Build history of the part. All positions in model axes, mm. A direction names the side the tool comes from. Round coordinates to 2 decimals unless told otherwise and drop trailing zeros. Order: outer loops, then holes, each group sorted by start corner. A loop starts at its lowest first (then second) coordinate and runs counter-clockwise, first axis right, second up. Notation, with made-up numbers: (-38, 37.25) -> (-17, 37.25) arc R21 cw to (-17, 68.25) -> close; hole circle Ø10 at (30.25, 57.25). An arc over 180 degrees is marked (long way). Write item = value, one per line.
from build123d import *

# Parameters (mm, degrees)
EXTRUDE_3_DEPTH = 10
EXTRUDE_START   = -12
EXTRUDE_4_DEPTH = 2
EXTRUDE_START_2 = 1
EXTRUDE_5_DEPTH = 1
SKETCH_2_R      = 5
SKETCH_2_R_2    = 3.5
EXTRUDE_6_DEPTH = 8
SKETCH_2_2_R    = 3.5
EXTRUDE_7_DEPTH = 7


# Read off the part's stored shape, not the designer's step: 凸台-拉伸4
with BuildPart() as part:
    # 草图1 → 凸台-拉伸3 (new body)
    with BuildSketch(Plane(origin=(0, 0, 0), x_dir=(1, 0, 0), z_dir=(0, 1, 0))):
        with BuildLine():
            Line((-8.229462415, 6.472103102), (-9.229462415, 7.472103102))
            ThreePointArc((-9.229462415, 7.472103102), (-9.371981305, 6.954608621), (-9.42, 6.42))
            Line((-9.42, 6.42), (-9.42, -6.42))
            ThreePointArc((-9.42, -6.42), (-9.371981305, -6.954608621), (-9.229462415, -7.472103102))
            Line((-9.229462415, -7.472103102), (-8.229462415, -6.472103102))
            ThreePointArc((-8.229462415, -6.472103102), (-8.371981305, -5.954608621), (-8.42, -5.42))
            Line((-8.42, -5.42), (-8.42, 5.42))
            ThreePointArc((-8.42, 5.42), (-8.371981305, 5.954608621), (-8.229462415, 6.472103102))
        make_face()
        with BuildLine():
            Line((-6.472103102, 8.229462415), (-7.472103102, 9.229462415))
            ThreePointArc((-7.472103102, 9.229462415), (-8.541320344, 8.541320344), (-9.229462415, 7.472103102))
            Line((-9.229462415, 7.472103102), (-8.229462415, 6.472103102))
            ThreePointArc((-8.229462415, 6.472103102), (-7.541320344, 7.541320344), (-6.472103102, 8.229462415))
        make_face()
        with BuildLine():
            ThreePointArc((7.472103102, 9.229462415), (6.954608621, 9.371981305), (6.42, 9.42))
            Line((6.42, 9.42), (-6.42, 9.42))
            ThreePointArc((-6.42, 9.42), (-6.954608621, 9.371981305), (-7.472103102, 9.229462415))
            Line((-7.472103102, 9.229462415), (-6.472103102, 8.229462415))
            ThreePointArc((-6.472103102, 8.229462415), (-5.954608621, 8.371981305), (-5.42, 8.42))
            Line((-5.42, 8.42), (5.42, 8.42))
            ThreePointArc((5.42, 8.42), (5.954608621, 8.371981305), (6.472103102, 8.229462415))
            Line((6.472103102, 8.229462415), (7.472103102, 9.229462415))
        make_face()
        with BuildLine():
            Line((-8.229462415, -6.472103102), (-9.229462415, -7.472103102))
            ThreePointArc((-9.229462415, -7.472103102), (-8.541320344, -8.541320344), (-7.472103102, -9.229462415))
            Line((-7.472103102, -9.229462415), (-6.472103102, -8.229462415))
            ThreePointArc((-6.472103102, -8.229462415), (-7.541320344, -7.541320344), (-8.229462415, -6.472103102))
        make_face()
        with BuildLine():
            ThreePointArc((6.42, -9.42), (6.954608621, -9.371981305), (7.472103102, -9.229462415))
            Line((7.472103102, -9.229462415), (6.472103102, -8.229462415))
            ThreePointArc((6.472103102, -8.229462415), (5.954608621, -8.371981305), (5.42, -8.42))
            Line((5.42, -8.42), (-5.42, -8.42))
            ThreePointArc((-5.42, -8.42), (-5.954608621, -8.371981305), (-6.472103102, -8.229462415))
            Line((-6.472103102, -8.229462415), (-7.472103102, -9.229462415))
            ThreePointArc((-7.472103102, -9.229462415), (-6.954608621, -9.371981305), (-6.42, -9.42))
            Line((-6.42, -9.42), (6.42, -9.42))
        make_face()
        with BuildLine():
            ThreePointArc((7.472103102, -9.229462415), (8.541320344, -8.541320344), (9.229462415, -7.472103102))
            Line((9.229462415, -7.472103102), (8.229462415, -6.472103102))
            ThreePointArc((8.229462415, -6.472103102), (7.541320344, -7.541320344), (6.472103102, -8.229462415))
            Line((6.472103102, -8.229462415), (7.472103102, -9.229462415))
        make_face()
        with BuildLine():
            ThreePointArc((9.42, 6.42), (9.371981305, 6.954608621), (9.229462415, 7.472103102))
            Line((9.229462415, 7.472103102), (8.229462415, 6.472103102))
            ThreePointArc((8.229462415, 6.472103102), (8.371981305, 5.954608621), (8.42, 5.42))
            Line((8.42, 5.42), (8.42, -5.42))
            ThreePointArc((8.42, -5.42), (8.371981305, -5.954608621), (8.229462415, -6.472103102))
            Line((8.229462415, -6.472103102), (9.229462415, -7.472103102))
            ThreePointArc((9.229462415, -7.472103102), (9.371981305, -6.954608621), (9.42, -6.42))
            Line((9.42, -6.42), (9.42, 6.42))
        make_face()
        with BuildLine():
            ThreePointArc((9.229462415, 7.472103102), (8.541320344, 8.541320344), (7.472103102, 9.229462415))
            Line((7.472103102, 9.229462415), (6.472103102, 8.229462415))
            ThreePointArc((6.472103102, 8.229462415), (7.541320344, 7.541320344), (8.229462415, 6.472103102))
            Line((8.229462415, 6.472103102), (9.229462415, 7.472103102))
        make_face()
    extrude(amount=-EXTRUDE_3_DEPTH)

    # 凸台-拉伸4 outline → 凸台-拉伸4 (add)
    with BuildSketch(Plane(origin=(0, 0, 0), x_dir=(1, 0, 0), z_dir=(0, 1, 0)).offset(EXTRUDE_START)):
        with BuildLine():
            Line((-9.42, 6.42), (-9.42, -6.42))
            ThreePointArc((-9.42, -6.42), (-8.541320344, -8.541320344), (-6.42, -9.42))
            Line((-6.42, -9.42), (6.42, -9.42))
            ThreePointArc((6.42, -9.42), (8.541320344, -8.541320344), (9.42, -6.42))
            Line((9.42, -6.42), (9.42, 6.42))
            ThreePointArc((9.42, 6.42), (8.541320344, 8.541320344), (6.42, 9.42))
            Line((6.42, 9.42), (-6.42, 9.42))
            ThreePointArc((-6.42, 9.42), (-8.541320344, 8.541320344), (-9.42, 6.42))
        make_face()
    extrude(amount=EXTRUDE_4_DEPTH)

    # 草图1<7> → 凸台-拉伸5 (add)
    with BuildSketch(Plane(origin=(0, 0, 0), x_dir=(1, 0, 0), z_dir=(0, 1, 0)).offset(EXTRUDE_START_2)):
        with BuildLine():
            Line((-8.229462415, 6.472103102), (-9.229462415, 7.472103102))
            ThreePointArc((-9.229462415, 7.472103102), (-9.371981305, 6.954608621), (-9.42, 6.42))
            Line((-9.42, 6.42), (-9.42, -6.42))
            ThreePointArc((-9.42, -6.42), (-9.371981305, -6.954608621), (-9.229462415, -7.472103102))
            Line((-9.229462415, -7.472103102), (-8.229462415, -6.472103102))
            ThreePointArc((-8.229462415, -6.472103102), (-8.371981305, -5.954608621), (-8.42, -5.42))
            Line((-8.42, -5.42), (-8.42, 5.42))
            ThreePointArc((-8.42, 5.42), (-8.371981305, 5.954608621), (-8.229462415, 6.472103102))
        make_face()
        with BuildLine():
            ThreePointArc((7.472103102, 9.229462415), (6.954608621, 9.371981305), (6.42, 9.42))
            Line((6.42, 9.42), (-6.42, 9.42))
            ThreePointArc((-6.42, 9.42), (-6.954608621, 9.371981305), (-7.472103102, 9.229462415))
            Line((-7.472103102, 9.229462415), (-6.472103102, 8.229462415))
            ThreePointArc((-6.472103102, 8.229462415), (-5.954608621, 8.371981305), (-5.42, 8.42))
            Line((-5.42, 8.42), (5.42, 8.42))
            ThreePointArc((5.42, 8.42), (5.954608621, 8.371981305), (6.472103102, 8.229462415))
            Line((6.472103102, 8.229462415), (7.472103102, 9.229462415))
        make_face()
        with BuildLine():
            ThreePointArc((9.42, 6.42), (9.371981305, 6.954608621), (9.229462415, 7.472103102))
            Line((9.229462415, 7.472103102), (8.229462415, 6.472103102))
            ThreePointArc((8.229462415, 6.472103102), (8.371981305, 5.954608621), (8.42, 5.42))
            Line((8.42, 5.42), (8.42, -5.42))
            ThreePointArc((8.42, -5.42), (8.371981305, -5.954608621), (8.229462415, -6.472103102))
            Line((8.229462415, -6.472103102), (9.229462415, -7.472103102))
            ThreePointArc((9.229462415, -7.472103102), (9.371981305, -6.954608621), (9.42, -6.42))
            Line((9.42, -6.42), (9.42, 6.42))
        make_face()
        with BuildLine():
            ThreePointArc((6.42, -9.42), (6.954608621, -9.371981305), (7.472103102, -9.229462415))
            Line((7.472103102, -9.229462415), (6.472103102, -8.229462415))
            ThreePointArc((6.472103102, -8.229462415), (5.954608621, -8.371981305), (5.42, -8.42))
            Line((5.42, -8.42), (-5.42, -8.42))
            ThreePointArc((-5.42, -8.42), (-5.954608621, -8.371981305), (-6.472103102, -8.229462415))
            Line((-6.472103102, -8.229462415), (-7.472103102, -9.229462415))
            ThreePointArc((-7.472103102, -9.229462415), (-6.954608621, -9.371981305), (-6.42, -9.42))
            Line((-6.42, -9.42), (6.42, -9.42))
        make_face()
    extrude(amount=-EXTRUDE_5_DEPTH)

    # 草图2 → 凸台-拉伸6 (add)
    with BuildSketch(Plane(origin=(0, -10, 0), x_dir=(1, 0, 0), z_dir=(0, 1, 0))):
        with Locations(Location((0, 0, 0), (0, 0, 270))):
            Circle(SKETCH_2_R)
        with Locations(Location((0, 0, 0), (0, 0, 270))):
            Circle(SKETCH_2_R_2, mode=Mode.SUBTRACT)
    extrude(amount=EXTRUDE_6_DEPTH)

    # 草图2<2> → 凸台-拉伸7 (add)
    with BuildSketch(Plane(origin=(0, -10, 0), x_dir=(1, 0, 0), z_dir=(0, 1, 0))):
        with Locations(Location((0, 0, 0), (0, 0, 270))):
            Circle(SKETCH_2_2_R)
    extrude(amount=EXTRUDE_7_DEPTH)


solid = part.part
Q1. Flat gauge pins, fed straight in: pin 1 (3 mm diameter, centred on x = 0, z = -1, fed in from +Y); pin 2 (5 mm diameter, centred on x = -0.5, z = 2.5, fed in from +Y); pin 3 (2 mm diameter, centred on x = 8, z = -8, fed in from +Y). Where does each tip first touch, or does it go through?
Check values:
pin_1 = -3
pin_2 = -2
pin_3 = 0
Q2. Cut at C-C, the plane z = 0. List the corners of the cut face in (x, y), and give its area (3 significant figures).
Check values:
outline = (-9.42, -12) -> (9.42, -12) -> (9.42, 1) -> (8.42, 1) -> (8.42, -10) -> (5, -10) -> (5, -2) -> (3.5, -2) -> (3.5, -3) -> (-3.5, -3) -> (-3.5, -2) -> (-5, -2) -> (-5, -10) -> (-8.42, -10) -> (-8.42, 1) -> (-9.42, 1) -> close
area = 133 mm²
Q3. Which spindle directions (+Z, -Z, +X, -X, +Y, -Y) get a long thin tool onto all of the face, cutting with end or side? Do faces 4 (the face through (6.98, 0.51, 8.74)), 5 (the face through (-6.965, 0.507, 8.722)), 6 (the face through (8, 0, 8)). Say none if no direction does.
Check values:
face_4 = +X, +Y
face_5 = -X, +Y
face_6 = +Y
Q4. Mould opens along X. For faces 1 (the face through (-4.88, -6.06, -1.08)), 2 (the face through (0, -5, -9.42)), 3 (the face through (6.965, 0.507, -8.722)) say: released by +X, released by -X, zero draft, split by the parting line, or undercut.
Check values:
face_1 = undercut
face_2 = zero draft
face_3 = released by +X
Q5. Cut at A-A, the plane y = -9. List the corners of the cut face in (x, z).
Check values:
outline = (-9.42, -6.42) arc R3 ccw to (-6.42, -9.42) -> (6.42, -9.42) arc R3 ccw to (9.42, -6.42) -> (9.42, 6.42) arc R3 ccw to (6.42, 9.42) -> (-6.42, 9.42) arc R3 ccw to (-9.42, 6.42) -> close; circle Ø10 at (0, 0); hole (-8.42, -5.42) arc R3 ccw to (-5.42, -8.42) -> (5.42, -8.42) arc R3 ccw to (8.42, -5.42) -> (8.42, 5.42) arc R3 ccw to (5.42, 8.42) -> (-5.42, 8.42) arc R3 ccw to (-8.42, 5.42) -> close
Q6. Cut at D-D, the plane x = 0. List the corners of the cut face in (y, z), and give its area (3 significant figures).
Check values:
outline = (-12, -9.42) -> (1, -9.42) -> (1, -8.42) -> (-10, -8.42) -> (-10, -5) -> (-2, -5) -> (-2, -3.5) -> (-3, -3.5) -> (-3, 3.5) -> (-2, 3.5) -> (-2, 5) -> (-10, 5) -> (-10, 8.42) -> (1, 8.42) -> (1, 9.42) -> (-12, 9.42) -> close
area = 133 mm²
Q7. Probe probe 1 along X at (y, z) = (-2.5, 0); probe 2 along X at (y, z) = (-1.75, 3.25); probe 3 along Z at (x, y) = (-4, -4.5). List the from-to ranges inside material, lowest first.
Check values:
probe_1 = -9.42 to -8.42, -5 to -3.5, 3.5 to 5, 8.42 to 9.42
probe_2 = -9.42 to -8.42, 8.42 to 9.42
probe_3 = -9.42 to -8.42, -3 to 3, 8.42 to 9.42
Q8. Cut at B-B, the plane y = 0.25. Give the number of separate pieces and of enclosed holes in the cut face, and give its area (3 significant figures).
Check values:
separate_pieces = 4
enclosed_holes = 0
area = 57.3 mm²
